Input: part model. Units: mm. Frame: model coordinates. A direction names the side the tool comes from. Round coordinates to 2 decimals unless told otherwise and drop trailing zeros. Loops run counter-clockwise (first coordinate to the right, second up) from the corner with the lowest first, then second, coordinate; pieces in that order, holes last.
1) Section A-A, the plane y = -14. Return loops of the section in (x, z).
2) Section C-C, the plane z = 34. State how many separate pieces and enclosed holes the cut face has, and give its area (3 significant figures).
3) Access query for faces 1 (the face through (20, 10, 70)), 2 (the face through (-15.5, -4, 70)). Directions: +Z, -Z, +X, -X, +Y, -Y. A direction counts if a zero-diameter tool reaches every point of the face in a straight line with its end or side. Return the directions, or none.
4) First-contact query: pin 1 (12 mm diameter, centred on x = 5.5, z = 35.5, fed in from -Y); pin 2 (0.8 mm diameter, centred on y = 19.5, z = 61.5, fed in from -X); pin 3 (0.5 mm diameter, centred on y = 3.5, z = 74.5, fed in from -X); pin 4 (0.8 mm diameter, centred on y = 19.5, z = 103.5, fed in from +X). Flat tips, straight axial feed; report the tip coordinate or a pass-through.
5) Ray query, line 1 along X through (y, z) = (-13, 88.5); line 2 along X through (y, z) = (-4, 48). Return the intervals inside material, ascending.
6) Draft query along Y for faces 3 (the face through (11, -20, 70)), 4 (the face through (11.69, 15, 70)), 5 (the face through (-5.385, 17, 70)). Return one class per face: pulls with the +Y half, pulls with the -Y half, needs draft (parallel to the pull), parting line crosses it, or undercut.
from build123d import *

# Parameters (mm, degrees)
BOSS_EXTRUDE1_DEPTH  = 142
MIRROR3_COPY_1_DEPTH = 142
MIRROR3_COPY_2_DEPTH = 142


with BuildPart() as part:
    # Sketch1 → Boss-Extrude1 (new body)
    with BuildSketch(Plane.XY):
        with BuildLine():
            Line((3.4, 0), (5.5, 0))
            Line((5.5, 0), (5.5, 4))
            Line((5.5, 4), (11.69, 10.19))
            Line((11.69, 10.19), (18.2, 10.19))
            Line((18.2, 10.19), (18.2, 5.265595036))
            Line((18.2, 5.265595036), (15.5, 5.265595036))
            Line((15.5, 5.265595036), (15.5, 2.965595036))
            Line((15.5, 2.965595036), (19, 2.965595036))
            Line((19, 2.965595036), (19, 3.965595036))
            Line((19, 3.965595036), (20, 3.965595036))
            Line((20, 3.965595036), (20, 15.5))
            ThreePointArc((20, 15.5), (18.681980515, 18.681980515), (15.5, 20))
            Line((15.5, 20), (6.385304712, 20))
            Line((6.385304712, 20), (6.385304712, 19))
            Line((6.385304712, 19), (5.385304712, 19))
            Line((5.385304712, 19), (5.385304712, 15.5))
            Line((5.385304712, 15.5), (7.685304712, 15.5))
            Line((7.685304712, 15.5), (7.685304712, 18.2))
            Line((7.685304712, 18.2), (10.19, 18.2))
            Line((10.19, 18.2), (10.19, 11.69))
            Line((10.19, 11.69), (4, 5.5))
            Line((4, 5.5), (0, 5.5))
            Line((0, 5.5), (0, 3.4))
            ThreePointArc((0, 3.4), (2.404163056, 2.404163056), (3.4, 0))
        make_face()
        with BuildLine():
            Line((18.5, 11.69), (18.5, 15.5))
            ThreePointArc((18.5, 15.5), (17.621320344, 17.621320344), (15.5, 18.5))
            Line((15.5, 18.5), (11.69, 18.5))
            Line((11.69, 18.5), (11.69, 11.69))
            Line((11.69, 11.69), (18.5, 11.69))
        make_face(mode=Mode.SUBTRACT)
    boss_extrude1 = extrude(amount=BOSS_EXTRUDE1_DEPTH)

    # Mirror1: Boss-Extrude1 across plane
    add(boss_extrude1.mirror(Plane.ZX))

    # Mirror2: Boss-Extrude1 across plane
    add(boss_extrude1.mirror(Plane(origin=(0, 0, 0), x_dir=(0, 0, 1), z_dir=(1, 0, 0))))

    # Mirror3 copy 1 sketch → Mirror3 copy 1 (add)
    with BuildSketch(Plane(origin=(0, 0, 0), x_dir=(-1, 0, 0), z_dir=(0, 0, 1))):
        with BuildLine():
            Line((3.4, 0), (5.5, 0))
            Line((5.5, 0), (5.5, 4))
            Line((5.5, 4), (11.69, 10.19))
            Line((11.69, 10.19), (18.2, 10.19))
            Line((18.2, 10.19), (18.2, 5.265595036))
            Line((18.2, 5.265595036), (15.5, 5.265595036))
            Line((15.5, 5.265595036), (15.5, 2.965595036))
            Line((15.5, 2.965595036), (19, 2.965595036))
            Line((19, 2.965595036), (19, 3.965595036))
            Line((19, 3.965595036), (20, 3.965595036))
            Line((20, 3.965595036), (20, 15.5))
            ThreePointArc((20, 15.5), (18.681980515, 18.681980515), (15.5, 20))
            Line((15.5, 20), (6.385304712, 20))
            Line((6.385304712, 20), (6.385304712, 19))
            Line((6.385304712, 19), (5.385304712, 19))
            Line((5.385304712, 19), (5.385304712, 15.5))
            Line((5.385304712, 15.5), (7.685304712, 15.5))
            Line((7.685304712, 15.5), (7.685304712, 18.2))
            Line((7.685304712, 18.2), (10.19, 18.2))
            Line((10.19, 18.2), (10.19, 11.69))
            Line((10.19, 11.69), (4, 5.5))
            Line((4, 5.5), (0, 5.5))
            Line((0, 5.5), (0, 3.4))
            ThreePointArc((0, 3.4), (2.404163056, 2.404163056), (3.4, 0))
        make_face()
        with BuildLine():
            Line((18.5, 11.69), (18.5, 15.5))
            ThreePointArc((18.5, 15.5), (17.621320344, 17.621320344), (15.5, 18.5))
            Line((15.5, 18.5), (11.69, 18.5))
            Line((11.69, 18.5), (11.69, 11.69))
            Line((11.69, 11.69), (18.5, 11.69))
        make_face(mode=Mode.SUBTRACT)
    extrude(amount=MIRROR3_COPY_1_DEPTH)

    # Mirror3 copy 2 sketch → Mirror3 copy 2 (add)
    with BuildSketch(Plane.XY):
        with BuildLine():
            Line((3.4, 0), (5.5, 0))
            Line((5.5, 0), (5.5, -4))
            Line((5.5, -4), (11.69, -10.19))
            Line((11.69, -10.19), (18.2, -10.19))
            Line((18.2, -10.19), (18.2, -5.265595036))
            Line((18.2, -5.265595036), (15.5, -5.265595036))
            Line((15.5, -5.265595036), (15.5, -2.965595036))
            Line((15.5, -2.965595036), (19, -2.965595036))
            Line((19, -2.965595036), (19, -3.965595036))
            Line((19, -3.965595036), (20, -3.965595036))
            Line((20, -3.965595036), (20, -15.5))
            ThreePointArc((20, -15.5), (18.681980515, -18.681980515), (15.5, -20))
            Line((15.5, -20), (6.385304712, -20))
            Line((6.385304712, -20), (6.385304712, -19))
            Line((6.385304712, -19), (5.385304712, -19))
            Line((5.385304712, -19), (5.385304712, -15.5))
            Line((5.385304712, -15.5), (7.685304712, -15.5))
            Line((7.685304712, -15.5), (7.685304712, -18.2))
            Line((7.685304712, -18.2), (10.19, -18.2))
            Line((10.19, -18.2), (10.19, -11.69))
            Line((10.19, -11.69), (4, -5.5))
            Line((4, -5.5), (0, -5.5))
            Line((0, -5.5), (0, -3.4))
            ThreePointArc((0, -3.4), (2.404163056, -2.404163056), (3.4, 0))
        make_face()
        with BuildLine():
            Line((18.5, -11.69), (18.5, -15.5))
            ThreePointArc((18.5, -15.5), (17.621320344, -17.621320344), (15.5, -18.5))
            Line((15.5, -18.5), (11.69, -18.5))
            Line((11.69, -18.5), (11.69, -11.69))
            Line((11.69, -11.69), (18.5, -11.69))
        make_face(mode=Mode.SUBTRACT)
    extrude(amount=MIRROR3_COPY_2_DEPTH)


solid = part.part
Final values:
1. outline: (-20, 0) - (-18.5, 0) - (-18.5, 142) - (-20, 142) - close; (-11.69, 0) - (-10.19, 0) - (-10.19, 142) - (-11.69, 142) - close; (10.19, 0) - (11.69, 0) - (11.69, 142) - (10.19, 142) - close; (18.5, 0) - (20, 0) - (20, 142) - (18.5, 142) - close
2. separate pieces: 1
2. enclosed holes: 5
2. area: 468 mm2
3. face 1: +Z, -Z, +X, +Y, -Y
3. face 2: +Z, -Z
4. pin 1: stops at y = -20
4. pin 2: stops at x = -18.2
4. pin 3: stops at x = -19
4. pin 4: stops at x = 18.2
5. line 1: x = -20 to -18.5, -11.69 to -10.19, 10.19 to 11.69, 18.5 to 20
5. line 2: x = -20 to -15.5, -5.5 to 5.5, 15.5 to 20
6. face 3: pulls with the -Y half
6. face 4: undercut
6. face 5: needs draft
